Solid Edge part; units mm, degrees
sketch "Sketch1" plane through (0, 0, 0) normal (0, -1, 0) x (1, 0, 0)
  line L0 (53.5, 0) -> (0, 0)
  line L1 (0, 0) -> (0, 15)
  line L2 (0, 15) -> (53.5, 15)
  line L3 (53.5, 15) -> (53.5, 0)
extrude "Protrusion1" add sketch "Sketch1" along normal blind 5
sketch "Sketch2" plane through (18.75, -5, 7.5) normal (0, -1, 0) x (1, 0, 0)
  line L0 (29.75, -7.5) -> (29.75, 7.5)
  line L1 (29.75, 7.5) -> (34.75, 7.5)
  line L2 (34.75, 7.5) -> (34.75, -7.5)
  line L3 (34.75, -7.5) -> (29.75, -7.5)
extrude "ExtrudedProtrusion_2" add sketch "Sketch2" along normal blind 30
sketch "Sketch3" plane through (18.75, 0, 7.5) normal (0, 1, 0) x (-1, 0, 0)
  line L0 (13.75, -7.5) -> (13.75, 7.5)
  line L1 (13.75, 7.5) -> (18.75, 7.5)
  line L2 (18.75, 7.5) -> (18.75, -7.5)
  line L3 (18.75, -7.5) -> (13.75, -7.5)
extrude "ExtrudedProtrusion_3" add sketch "Sketch3" along normal blind 15
sketch "Sketch4" plane through (53.5, -17.5, 7.5) normal (1, 0, 0) x (0, 1, 0)
  circle A0 centre (-2.5, 0) radius 4
extrude "Cutout1" cut sketch "Sketch4" against normal through all
sketch "Sketch5" plane through (0, 5, 7.5) normal (-1, 0, 0) x (0, -1, 0)
  circle A0 centre (-3, 0) radius 4
extrude "Cutout2" cut sketch "Sketch5" against normal through all
fillet "Round1" radius 7 2 edges at (2.5, 15, 15) (2.5, 15, 0)
hole "Hole_1" at (0, 8, 7.5) direction (1, 0, 0) diameter 8.4 end up to next
hole "Hole_2" at (53.5, -20, 7.5) direction (-1, 0, 0) diameter 8.4 end up to next
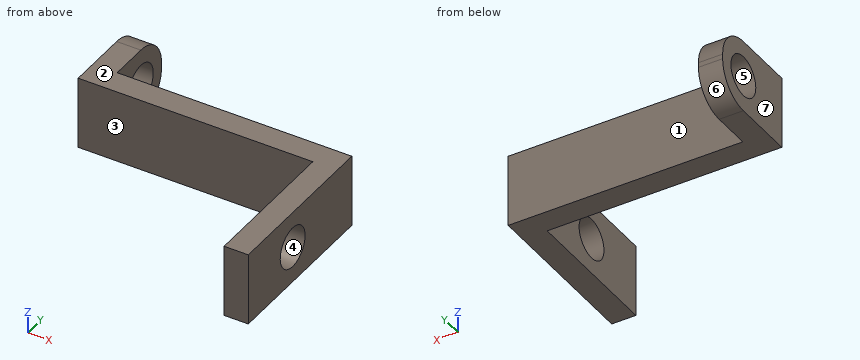
Source: CAD feature listing. Evaluate the final solid. Frame: model axes, mm. Face numbers are marked on the shaded views. A direction names the side the tool comes from. Give positions to 0.01 mm unless a question says otherwise; leave off trailing zeros. Write each loop counter-clockwise with the first axis right and the second up, starting at its lowest first coordinate (ties: lowest second). Pieces come first, ordered by that corner, then holes. Notation, with made-up numbers: M 82,72 L 88,72 A25 ccw 88,86 Z; hole C 81,-27 d2. An arc over 180 degrees is marked long. Return JSON: item names as keys, results as strings. Group by question number.
1) Draft query along Z for the marked faces 4, 5, 6 and 7. Return one class per face: released by +Z, released by -Z, zero draft, split by the parting line, or undercut.
2) First-contact query: pin 1 Ø1.5 at (x, z) = (26.5, 6) entering from +Y; pin 2 Ø6 at (y, z) = (3.5, 4.5) entering from +X; pin 3 Ø6 at (x, z) = (31.5, 13) entering from -Y; pin 4 Ø6 at (x, y) = (32, -9) entering from +Z. Flat tips, straight axial feed; report the tip coordinate or a pass-through.
3) Cut plane A-A, the plane y = -20. Output: boundary loops of the cut face in (x, z), then the cut area to 3 significant figures.
4) Cut plane C-C, the plane x = 16. Output: boundary loops of the cut face in (y, z).
5) Set-up query: the marked faces 1, 2 and 3. Return all of +Z, -Z, +X, -X, +Y, -Y with unobstructed straight access to the full face (end or side cutting, diameter ignored); none if empty.
6) Ray query, L1, parallel to Y at x = 1.45, z = 7.5; L2, parallel to Y at x = 49, z = 7.25; L3, parallel to Z at x = 3.65, y = 8. Return the intervals inside material, ascending.
7) Cut plane B-B, the plane z = 11. Output: boundary loops of the cut face in (x, y), then the cut area to 3 significant figures.
8) Cut plane D-D, the plane y = -12.5. Output: boundary loops of the cut face in (x, z).
Data:
{
 "1": {"face 4": "undercut", "face 5": "undercut", "face 6": "released by -Z", "face 7": "zero draft"},
 "2": {"pin 1": "stops at y = 0", "pin 2": "stops at x = 5", "pin 3": "stops at y = -5", "pin 4": "passes through"},
 "3": {"outline": "M 48.5,0 L 53.5,0 L 53.5,3.3 L 48.5,3.3 Z; M 48.5,11.7 L 53.5,11.7 L 53.5,15 L 48.5,15 Z", "area": "33.0 mm²"},
 "4": {"outline": "M -5,0 L 0,0 L 0,15 L -5,15 Z"},
 "5": {"face 1": "+Z, -Z, +X, +Y", "face 2": "+Z, +X, -X, +Y, -Y", "face 3": "+Z, -Z, -X, -Y"},
 "6": {"L1": "y = -5 to 3.8, 12.2 to 15", "L2": "y = -35 to -24.19, -15.81 to 0", "L3": "z = 0 to 3.3, 11.7 to 15"},
 "7": {"outline": "M 0,-5 L 48.5,-5 L 48.5,-17.68 L 53.5,-17.68 L 53.5,0 L 5,0 L 5,5.68 L 0,5.68 Z; M 0,10.32 L 5,10.32 L 5,14.32 L 0,14.32 Z; M 48.5,-35 L 53.5,-35 L 53.5,-22.32 L 48.5,-22.32 Z", "area": "443 mm²"},
 "8": {"outline": "M 48.5,0 L 53.5,0 L 53.5,15 L 48.5,15 Z"}
}
